from build123d import *

# Parameters (mm, degrees)
BOSS_EXTRUDE1_DEPTH      = 3.175
BOSS_EXTRUDE1_DEPTH_BACK = 3.175
CUT_EXTRUDE3_DEPTH       = 206.528461822
CUT_EXTRUDE5_DEPTH       = 206.528461822
CUT_EXTRUDE6_DEPTH       = 6.35


with BuildPart() as part:
    # Sketch1 → Boss-Extrude1 (new, two sides: drawn at the far end of the back side and taken through both)
    with BuildSketch(Plane.XY.offset(-BOSS_EXTRUDE1_DEPTH_BACK)):
        with BuildLine():
            Line((-95.480291898, -80.706386575), (-95.480291898, -131.085242165))
            Line((-95.480291898, -131.085242165), (-95.480291898, -132.672742165))
            Line((-95.480291898, -132.672742165), (-120.480291898, -132.672742165))
            Line((-120.480291898, -132.672742165), (-120.480291898, -131.085242165))
            Line((-120.480291898, -131.085242165), (-120.480291898, -64.018285781))
            ThreePointArc((-120.480291898, -64.018285781), (-115.755703828, -49.392703021), (-103.367678212, -40.295108567))
            Line((-103.367678212, -40.295108567), (119.519708102, 33.809591006))
            Line((119.519708102, 33.809591006), (119.519708102, 8.809591006))
            Line((119.519708102, 8.809591006), (-78.367678212, -56.983209361))
            ThreePointArc((-78.367678212, -56.983209361), (-90.755703828, -66.080803815), (-95.480291898, -80.706386575))
        make_face()
    extrude(amount=BOSS_EXTRUDE1_DEPTH + BOSS_EXTRUDE1_DEPTH_BACK)

    # Sketch2 → Cut-Extrude3 (cut, through all)
    with BuildSketch(Plane.XZ.offset(132.672742165)):
        Polygon((-120.480291898, 0), (-120.480291898, 3.175), (-118.647204793, 3.175), align=None)
    cut_extrude3 = extrude(amount=-CUT_EXTRUDE3_DEPTH, mode=Mode.SUBTRACT)

    # Mirror3: Cut-Extrude3 across plane
    add(cut_extrude3.mirror(Plane.XY), mode=Mode.SUBTRACT)

    # Sketch3 → Cut-Extrude5 (cut, through all)
    with BuildSketch(Plane.XZ.offset(132.672742165)):
        Polygon((119.519708102, 3.175), (114.020446788, 3.175), (119.519708102, 0), align=None)
    cut_extrude5 = extrude(amount=-CUT_EXTRUDE5_DEPTH, mode=Mode.SUBTRACT)

    # Mirror4: Cut-Extrude5 across plane
    add(cut_extrude5.mirror(Plane.XY), mode=Mode.SUBTRACT)

    # Sketch6 → Cut-Extrude6 (cut)
    with BuildSketch(Plane.XY.offset(3.175)):
        Polygon((33.546459297, -19.774448133), (38.29109474, -18.19697087), (35.769730347, -16.267373348), (31.025094904, -17.844850611), align=None)
    extrude(amount=-CUT_EXTRUDE6_DEPTH, mode=Mode.SUBTRACT)


solid = part.part
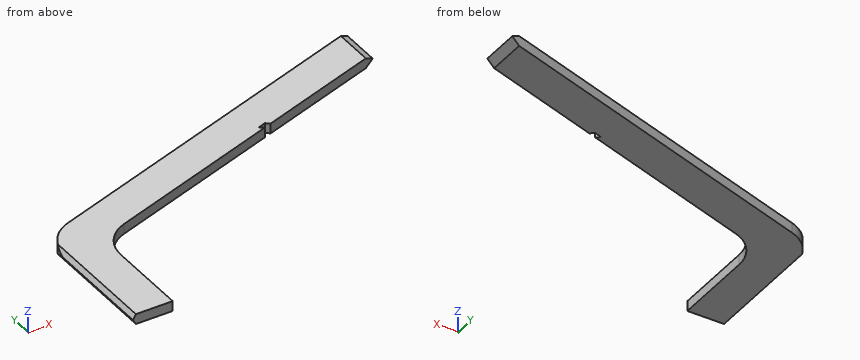
The listing builds one solid part. Answer for the finished solid, in the listing's coordinates (mm). Round coordinates to 2 decimals unless told otherwise and drop trailing zeros. Write each loop counter-clockwise with the first axis right and the second up, starting at its lowest first coordinate (ties: lowest second). Pieces come first, ordered by that corner, then holes. Notation, with made-up numbers: M 89,37.25 L 96,37.25 A22 cw 96,71.25 Z; hole C 32,76 d5. An arc over 180 degrees is marked long. Write each question's results on one line, items separated by ' | '. Start each with the question number.
Item 1: Find section C-C on x = -86.5. Write down the section's boundary in (y, z) (3 decimals), and give its area (3 significant figures).
Item 2: Find section B-B on z = 1.25. Write down the section's boundary in (x, y).
Item 3: Straight lines are drawn through the part: probe 1 along Y at (x, z) = (82, -1.75); probe 2 along X at (y, z) = (-118.5, 0.25); probe 3 along Y at (x, z) = (-24, 0.5). For each, find the intervals that lie inside material, in ascending order.
Item 4: Given pin 1 Ø3 at (y, z) = (-117.5, 1) entering from +X; pin 2 Ø1 at (y, z) = (-113, 1) entering from -X, each flat-ended and moving along its own axis, determine where each tip first touches the part or whether it passes through.
Item 5: Find section D-D on y = 12. Write down the section's boundary in (x, z) (3 decimals), and give its area (3 significant figures).
Item 6: Find section A-A on y = -89. Write down the section's boundary in (x, z) (3 decimals).
Answer block:
1) outline: M -61.513,-3.175 L -34.687,-3.175 L -34.687,3.175 L -61.513,3.175 Z | area: 170 mm²
2) outline: M -119.76,-132.67 L -95.48,-132.67 L -95.48,-80.71 A25 cw -78.37,-56.98 L 33.55,-19.77 L 31.03,-17.84 L 35.77,-16.27 L 38.29,-18.2 L 117.35,8.09 L 117.35,33.09 L -103.37,-40.3 A25 ccw -119.76,-58.05 Z
3) probe 1: y = -3.66 to 21.34 | probe 2: x = -120.34 to -95.48 | probe 3: y = -38.91 to -13.91
4) pin 1: stops at x = -95.48 | pin 2: stops at x = -120.19
5) outline: M 53.922,-3.175 L 114.02,-3.175 L 119.52,0 L 114.02,3.175 L 53.922,3.175 Z | area: 399 mm²
6) outline: M -120.48,0 L -118.647,-3.175 L -95.48,-3.175 L -95.48,3.175 L -118.647,3.175 Z
